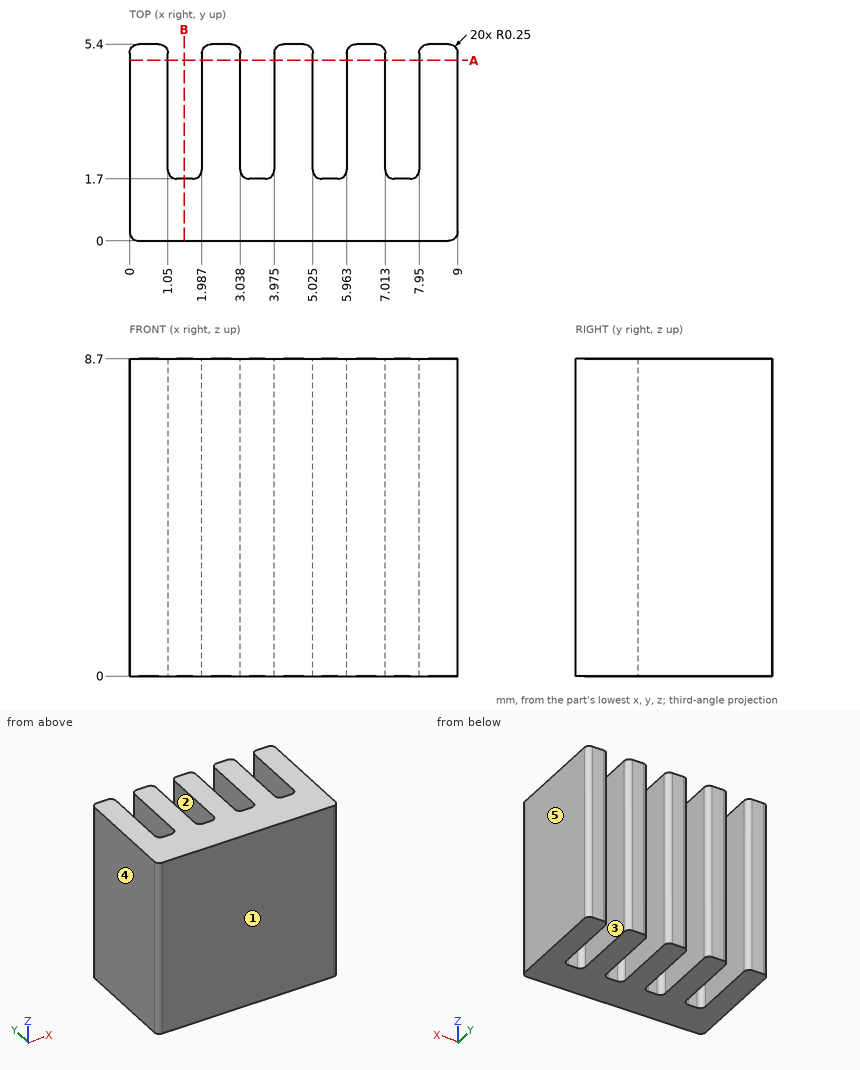
Could you check a few things on this drawing? It's one solid part, dimensions in mm from its lowest x, y, z. A direction names the side the tool comes from. Coordinates: 2 decimals unless noted, no trailing zeros. Order: outer loops, then holes, each group sorted by start corner. A loop starts at its lowest first (then second) coordinate and runs counter-clockwise, first axis right, second up.
1. If we section it at B-B (x = 1.5): Please give me the cut outline in (y, z), then the cut area to 3 significant figures.
2. Thinking about a two-plate mould opening in X: for the marked faces 3, 4 and 5, which applies, +X half, -X half, draft (parallel to the pull), parting line (faces both ways), or undercut?
3. If we section it at A-A (y = 4.95): Give the number of separate pieces and of enclosed holes in the cut face.
4. I'm going to push flat-ended pins straight in: pin 1 (0.5 mm diameter, centred on x = 3.5, z = 3, fed in from +Y); pin 2 (1 mm diameter, centred on y = 3.5, z = 4.5, fed in from -X). Where does each tip first touch, or does it pass through?
5. I need wall thicknesses on line 1 (X direction, y = 1.8, z = 4.25) (1 decimal); line 2 (Y direction, x = 3.25, z = 6.5). Which ranges of each line are inside material? Lowest first, please.
6. For the marked faces 1 and 2, which set-ups out of +Z, -Z, +X, -X, +Y, -Y let a thin tool reach every point of the face, with its end or its side?
Entries:
1. outline: (0, 0) - (1.7, 0) - (1.7, 8.7) - (0, 8.7) - close
1. area: 14.8 mm2
2. face 3: undercut
2. face 4: -X half
2. face 5: +X half
3. separate pieces: 5
3. enclosed holes: 0
4. pin 1: stops at y = 1.7
4. pin 2: stops at x = 0
5. line 1: x = 0 to 1.1, 1.9 to 3.1, 3.9 to 5.1, 5.9 to 7.1, 7.9 to 9
5. line 2: y = 0 to 1.7
6. face 1: +Z, -Z, +X, -X, -Y
6. face 2: +Z, -Z, +Y
